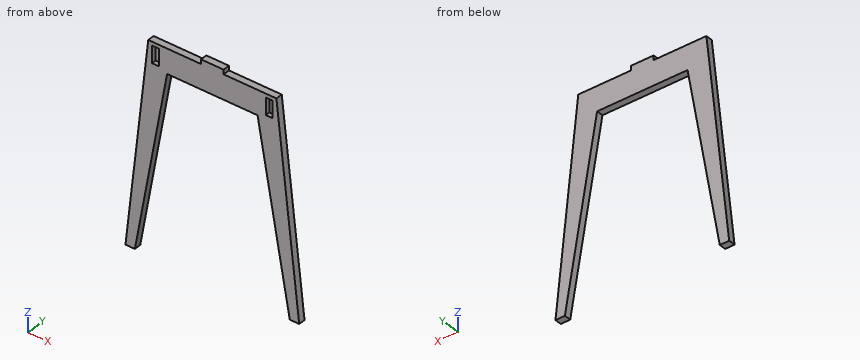
```python
from build123d import *

# Parameters (mm, degrees)
PAD_DEPTH    = 18
SKETCH001_W  = 18
SKETCH001_H  = 45
POCKET_DEPTH = 12


with BuildPart() as part:
    # Sketch → Pad (new body)
    with BuildSketch(Plane.XZ):
        Polygon((-230.518586, 0), (-170, 550), (-30, 550), (-30, 562), (30, 562), (30, 550), (170, 550), (230.518586, 0), (205.518586, 0), (120, 485), (-120, 485), (-205.518586, 0), align=None)
    extrude(amount=PAD_DEPTH)

    # Sketch001 → Pocket (cut)
    with BuildSketch(Plane.XZ.offset(18)):
        with Locations((-151, 517.5)):
            Rectangle(SKETCH001_W, SKETCH001_H)
        with Locations((151, 517.5)):
            Rectangle(SKETCH001_W, SKETCH001_H)
    extrude(amount=-POCKET_DEPTH, mode=Mode.SUBTRACT)


solid = part.part
```
Part model, mm, in its own coordinate system. Give positions to 0.01 mm unless a question says otherwise; leave off trailing zeros. Write each loop counter-clockwise with the first axis right and the second up, starting at its lowest first coordinate (ties: lowest second). Pieces come first, ordered by that corner, then holes. Notation, with made-up numbers: (88, 12.25) -> (114, 12.25) arc R19 ccw to (114, 37.25) -> close; hole circle Ø2 at (38, 66). An arc over 180 degrees is marked (long way). Put each result on its own line as item: value. Start each with the question number.
Item 1: Wall check: L1, parallel to X at y = -0.75, z = 264; L2, parallel to Z at x = 48.5, y = -10.5; L3, parallel to X at y = -15.5, z = 260. Give the ranges that are in metal, low to high. Write a range as [from, to].
Item 2: Cut at A-A (y = -10.75). List the corners of the cut face in (x, z), then the cut area to 3 significant figures.
Item 3: Cut at D-D (x = 10). List the corners of the cut face in (y, z), then the cut area to 3 significant figures.
Item 4: Pin check, flat tips, straight feed: pin 1 Ø4 at (x, y) = (93.5, -12) entering from -Z; pin 2 Ø3.5 at (y, z) = (-14, 514.5) entering from +X; pin 3 Ø3.5 at (y, z) = (-7, 555.5) entering from -X. Stop position of each tip, or through.
Item 5: Cut at B-B (z = 462.5). List the corners of the cut face in (x, y).
Item 6: Cut at C-C (z = 113). List the corners of the cut face in (x, y), then the cut area to 3 significant figures.
Answer list:
1. L1: x = [-201.47, -158.97], [158.97, 201.47]
1. L2: z = [485, 550]
1. L3: x = [-201.91, -159.67], [159.67, 201.91]
2. outline: (-230.52, 0) -> (-205.52, 0) -> (-120, 485) -> (120, 485) -> (205.52, 0) -> (230.52, 0) -> (170, 550) -> (30, 550) -> (30, 562) -> (-30, 562) -> (-30, 550) -> (-170, 550) -> close; hole (-160, 495) -> (-142, 495) -> (-142, 540) -> (-160, 540) -> close; hole (142, 495) -> (160, 495) -> (160, 540) -> (142, 540) -> close
2. area: 61,500 mm2
3. outline: (-18, 485) -> (0, 485) -> (0, 562) -> (-18, 562) -> close
3. area: 1,390 mm2
4. pin 1: stops at z = 485
4. pin 2: stops at x = 174.1
4. pin 3: stops at x = -30
5. outline: (-179.63, -18) -> (-123.97, -18) -> (-123.97, 0) -> (-179.63, 0) -> close; (123.97, -18) -> (179.63, -18) -> (179.63, 0) -> (123.97, 0) -> close
6. outline: (-218.08, -18) -> (-185.59, -18) -> (-185.59, 0) -> (-218.08, 0) -> close; (185.59, -18) -> (218.08, -18) -> (218.08, 0) -> (185.59, 0) -> close
6. area: 1,170 mm2
